Build history of the part. All positions in model axes, mm. A direction names the side the tool comes from. Round coordinates to 2 decimals unless told otherwise and drop trailing zeros. Write each loop counter-clockwise with the first axis right and the second up, starting at its lowest first coordinate (ties: lowest second). Pieces come first, ordered by that corner, then holes. Notation, with made-up numbers: (26, -1) -> (75, -1) arc R24 ccw to (75, 20) -> close; hole circle Ø9 at (24, 76.5). An arc over 180 degrees is marked (long way). Answer as CSV lines item,"result".
Autodesk Inventor part; units mm, degrees
ref_plane "YZ Plane" through (0, 0, 0) normal (1, 0, 0) x (0, 1, 0)
ref_plane "XZ Plane" through (0, 0, 0) normal (0, 1, 0) x (-1, 0, 0)
ref_plane "XY Plane" through (0, 0, 0) normal (0, 0, 1) x (1, 0, 0)
sketch "Sketch1" plane through (0, 0, 0) normal (0, 1, 0) x (-1, 0, 0)
  line L0 (0, 0) -> (24, 0)
  line L1 (24, 0) -> (24, -24)
  line L2 (24, -24) -> (0, -24)
  line L3 (0, -24) -> (0, 0)
  dimension "d0" = 24
  dimension "d1" = 24
extrude "Extrusion1" add sketch "Sketch1" along normal blind 5
sketch "Sketch2" plane through (0, 0, 0) normal (0, -1, 0) x (1, 0, 0)
  line L0 (0, 0) -> (0, -3)
  line L1 (0, 0) -> (0, -24)
  line L2 (-24, -24) -> (-24, 0)
  line L3 (0, -3) -> (-24, -3)
  line L4 (-24, -3) -> (-24, -5)
  line L5 (-24, -5) -> (0, -5)
  line L6 (0, -5) -> (0, -3)
  dimension "d4" = 3
  dimension "d5" = 2
extrude "Extrusion2" add sketch "Sketch2" along normal blind 6
sketch "Sketch3" plane through (-24, 0, -3) normal (0, 0, 1) x (1, 0, 0)
  line L0 (24, -6) -> (0, -6)
  line L1 (0, -6) -> (24, -6)
  line L2 (12, -6) -> (12, -5)
  line L3 (12, -5) -> (12, -2.875)
  circle A0 centre (12, -2.875) radius 2.125
  point P0 (24, 0)
  dimension "d8" = 1
  dimension "d11" = 2.125
  dimension "d12" = 4.25
sketch "Sketch4" plane through (0, 5, 0) normal (0, 1, 0) x (1, 0, 0)
  line L0 (-24, 24) -> (0, 24)
  line L1 (0, 24) -> (0, 26)
  line L2 (0, 26) -> (-24, 26)
  line L3 (-24, 26) -> (-24, 24)
  point P0 (0, 0)
  dimension "d13" = 2
extrude "Extrusion3" add sketch "Sketch4" against normal blind 11
sketch "Sketch5" plane through (0, 5, 0) normal (0, 1, 0) x (1, 0, 0)
  line L0 (-24, 5) -> (-24, 24)
  line L1 (0, 3) -> (-24, 3)
  line L2 (-24, 3) -> (-24, 9)
  line L3 (-24, 9) -> (0, 9)
  line L4 (0, 9) -> (0, 3)
  point P0 (0, 0)
  dimension "d16" = 6
extrude "Extrusion4" add sketch "Sketch5" along normal blind 10
extrude "Extrusion6" cut sketch "Sketch3" against normal through all
pattern_linear "Rectangular Pattern1" count 3 spacing 6 along (-1, 0, 0) of "Extrusion6" first direction both ways yes
sketch "Sketch7" plane through (0, 5, -26) normal (0, 0, -1) x (-1, 0, 0)
  circle A0 centre (18, -7.875) radius 2.125
  line L0 (15.875, -7.875) -> (14.125, -7.875)
  circle A1 centre (12, -7.875) radius 2.125
  circle A2 centre (6, -7.875) radius 2.125
  line L1 (8.125, -7.875) -> (9.875, -7.875)
  line L2 (15, -7.875) -> (15, -11)
  line L3 (24, -11) -> (0, -11)
  line L4 (9, -7.875) -> (9, -5)
  line L5 (0, -5) -> (24, -5)
  line L6 (15, -11) -> (9, -11)
  line L7 (9, -11) -> (9, -5)
  line L8 (9, -5) -> (15, -5)
  line L9 (15, -5) -> (15, -11)
sketch "Sketch8" plane through (-24, 0, -3) normal (0, 0, 1) x (1, 0, 0)
  circle A0 centre (18, -2.875) radius 2.125
  line L0 (15.875, -2.875) -> (14.125, -2.875)
  circle A1 centre (12, -2.875) radius 2.125
  line L1 (9.875, -2.875) -> (8.125, -2.875)
  circle A2 centre (6, -2.875) radius 2.125
  line L2 (0, -6) -> (24, -6)
  line L3 (9, -6) -> (9, 0)
  line L4 (24, 0) -> (0, 0)
  line L5 (15, -6) -> (15, 0)
  line L6 (15, -6) -> (9, -6)
  line L7 (9, -6) -> (9, 0)
  line L8 (9, 0) -> (15, 0)
  line L9 (15, 0) -> (15, -6)
extrude "Extrusion7" cut sketch "Sketch8" against normal blind 2 contours L5 L2 L3 L1 A1 L0 | L0 A1 L1 L3 L4 L5
sketch "Sketch9" plane through (0, -6, -3) normal (0, 0, 1) x (1, 0, 0)
  line L0 (-9, 6) -> (-9, 0)
  line L1 (-9, 0) -> (0, 0)
  circle A0 centre (-6, 3.125) radius 2.125
  line L2 (-15, 0) -> (-15, 6)
  line L3 (-24, 0) -> (0, 0)
  circle A1 centre (-18, 3.125) radius 2.125
  line L4 (-9, 0) -> (-7.5, 0)
  line L5 (-15, 0) -> (-16.5, 0)
  line L6 (-9, 0) -> (-9, 1.3884)
  arc A2 (-9, 1.3884) -> (-7.5, 0) centre (-6, 3.125) ccw
  line L7 (-15, 0) -> (-15, 1.3884)
  arc A3 (-16.5, 0) -> (-15, 1.3884) centre (-18, 3.125) ccw
  point P0 (0, 6)
  dimension "d33" = 1.5
  dimension "d34" = 1.5
extrude "Extrusion8" cut sketch "Sketch9" against normal blind 2 contours A2 L1 L0 | L3 A3 L2
sketch "Sketch10" plane through (0, 0, 0) normal (1, 0, 0) x (0, 0, -1)
  line L0 (9, 5) -> (19, 5)
  line L1 (19, 5) -> (19, 15)
  line L2 (19, 15) -> (9, 15)
  line L3 (9, 15) -> (9, 5)
  point P0 (0, 0)
  dimension "d37" = 10
extrude "Extrusion9" add sketch "Sketch10" against normal blind 24
sketch "Sketch11" plane through (0, 15, 0) normal (0, 1, 0) x (1, 0, 0)
  line L0 (0, 5) -> (0, 19)
  line L1 (0, 19) -> (-24, 19)
  line L2 (-24, 19) -> (-24, 3)
  line L3 (-24, 3) -> (0, 3)
  line L4 (0, 3) -> (0, 19)
  point P0 (0, 0)
  point P1 (-24, 5)
extrude "Extrusion10" add sketch "Sketch11" along normal blind 10
sketch "Sketch13" plane through (0, 0, 0) normal (1, 0, 0) x (0, 0, -1)
  line L0 (3, 25) -> (19, 25)
  line L1 (19, 25) -> (19, 5)
  line L2 (19, 5) -> (3, 5)
  line L3 (3, 5) -> (3, 25)
  point P0 (0, 0)
extrude "Extrusion11" add sketch "Sketch13" along normal blind 12
sketch "Sketch14" plane through (-24, 5, -3) normal (0, 0, 1) x (1, 0, 0)
  line L0 (24, 0) -> (24, 20)
  line L1 (0, 20) -> (36, 20)
  line L2 (24, 10) -> (32, 10)
  circle A0 centre (28, 10) radius 3.75
  point P0 (24, -5)
  dimension "d44" = 8
  dimension "d45" = 7.5
extrude "Extrusion12" add sketch "Sketch14" along normal blind 20
sketch "Sketch15" plane through (-24, 0, 0) normal (-1, 0, 0) x (0, 0, 1)
  line L0 (-3, 25) -> (0, 25)
  line L1 (0, 25) -> (0, 5)
  line L2 (0, 5) -> (-3, 5)
  line L3 (-3, 5) -> (-3, 25)
  point P0 (0, 0)
extrude "Extrusion13" add sketch "Sketch15" against normal blind 36
sketch "Sketch16" plane through (-24, 0, -3) normal (-1, 0, 0) x (0, 0, 1)
  line L0 (3, 25) -> (-16, 25)
  line L1 (-16, 25) -> (-16, 5)
  line L2 (-16, 5) -> (3, 5)
  line L3 (3, 5) -> (3, 25)
  point P0 (3, 0)
extrude "Extrusion14" add sketch "Sketch16" along normal blind 12
sketch "Sketch17" plane through (-24, 0, 0) normal (0, 0, 1) x (1, 0, 0)
  line L0 (-12, 25) -> (-12, 5)
  line L1 (-12, 15) -> (-4, 15)
  circle A0 centre (-4, 15) radius 3.9
  point P0 (24, 0)
  dimension "d52" = 8
  dimension "d53" = 7.8
extrude "Extrusion15" add sketch "Sketch17" along normal blind 20
sketch "Sketch18" plane through (-24, 0, 0) normal (0, 0, 1) x (1, 0, 0)
  line L0 (24, 5) -> (36, 5)
  line L1 (36, 5) -> (36, 25)
  line L2 (36, 25) -> (24, 25)
  line L3 (24, 25) -> (24, 5)
  point P0 (24, 0)
extrude "Extrusion16" cut sketch "Sketch18" along normal through all both and the other way through all
properties part number "RearBearingMount"
1. Cut at A-A, the plane x = -12. Write the cut outline in (y, z).
Results found:
outline,"(-6, -26) -> (-5, -26) -> (-5, -24) -> (-6, -24) -> close; (-0.75, -26) -> (5, -26) -> (5, -19) -> (25, -19) -> (25, 0) -> (0, 0) -> (0, -24) -> (-0.75, -24) -> close"
2. Cut at B-B, the plane z = -1.5. Write the cut outline in (x, y).
Results found:
outline,"(-36, 5) -> (-24, 5) -> (-24, 0) -> (0, 0) -> (0, 25) -> (-36, 25) -> close"
3. Cut at C-C, the plane x = -3. Write the cut outline in (y, z).
Results found:
outline,"(-6, -26) -> (5, -26) -> (5, -19) -> (25, -19) -> (25, 0) -> (0, 0) -> (0, -3) -> (-6, -3) -> (-6, -5) -> (0, -5) -> (0, -24) -> (-6, -24) -> close"
4. Drop flat-ended pins along their axis: pin 1 Ø7 at (x, z) = (-13.5, -16) entering from -Y; pin 2 Ø5 at (x, z) = (-22.5, 15) entering from +Y; pin 3 Ø10 at (y, z) = (17.5, 7.5) entering from +X. Give the stop position or say it passes through.
Results found:
pin 1,"stops at y = 0"
pin 2,"stops at y = 17.49"
pin 3,"stops at x = -24.1"
5. Cut at D-D, the plane y = 15. Write the cut outline in (x, z).
Results found:
outline,"(-36, -19) -> (0, -19) -> (0, 0) -> (-24.1, 0) -> (-24.1, 20) -> (-31.9, 20) -> (-31.9, 0) -> (-36, 0) -> close"
6. Mould opens along X. For faces 1 (the flat face through (-15, -2, -4)), 2 (the flat face through (0, 13, -10)), 3 (the flat face through (-12, 5, -23)), 4 (the flat face through (-24, 2, -13)) say: +X half, -X half, draft (parallel to the pull), parting line (faces both ways), or undercut.
Results found:
face 1,"undercut"
face 2,"+X half"
face 3,"draft"
face 4,"-X half"
7. Which spindle directions (+Z, -Z, +X, -X, +Y, -Y) get a long thin tool onto all of the face, cutting with end or side? Do faces 5 (the flat face through (-21, -3, -5)), 6 (the flat face through (-20.4, -3, -3)), 7 (the flat face through (-28, 15, 20)), 8 (the flat face through (-30, 5, -10)), 9 (the flat face through (-9, -2, -4)). Say none if no direction does.
Results found:
face 5,"+X, -X, -Y"
face 6,"+Z, +X, -X, -Y"
face 7,"+Z, +X, -X, +Y, -Y"
face 8,"+Z, -Z, -X, -Y"
face 9,"+Z, -Y"
8. Probe line 1 along Y through (x, z) = (-18, -4); line 2 along Y through (x, z) = (-12, -25.4); line 3 along Y through (x, z) = (-24.5, -12). List the from-to ranges inside material, lowest first.
Results found:
line 1,"y = -6 to -5, -0.75 to 25"
line 2,"y = -6 to -5, -0.75 to 5"
line 3,"y = 5 to 25"
